Verification items for the finished model (mm, model axes). Coordinates: 2 decimals unless noted, no trailing zeros. Write each loop counter-clockwise with the first axis right and the second up, starting at its lowest first coordinate (ties: lowest second). Pieces come first, ordered by that corner, then holes. Notation, with made-up numbers: (77, -7) -> (132, -7) arc R24 ccw to (132, 26) -> close; hole circle Ø1 at (36.25, 51). An arc over 180 degrees is marked (long way). Answer in a Markdown table with one row per item.
```python
from build123d import *

# Parameters (mm, degrees)
F1_DEPTH = 12.7
F2_R     = 25.4
F3_DEPTH = 25.401


with BuildPart() as f1:
    # F0 (on Front) → F1 (new body, symmetric)
    with BuildSketch(Plane.XZ):
        with BuildLine():
            Line((952.5, 50.8), (-952.5, 50.8))
            ThreePointArc((-952.5, 50.8), (-1003.3, 0), (-952.5, -50.8))
            Line((-952.5, -50.8), (952.5, -50.8))
            ThreePointArc((952.5, -50.8), (1003.3, 0), (952.5, 50.8))
        make_face()
    extrude(amount=F1_DEPTH, both=True)

    # F2 (on face) → F3 (cut, through all)
    with BuildSketch(Plane.XZ.offset(12.7)):
        with Locations((-952.5, 0)):
            Circle(F2_R)
        with Locations((952.5, 0)):
            Circle(F2_R)
        with Locations((-317.5, 0)):
            Circle(F2_R)
    extrude(amount=-F3_DEPTH, mode=Mode.SUBTRACT)


solid = f1.part
```
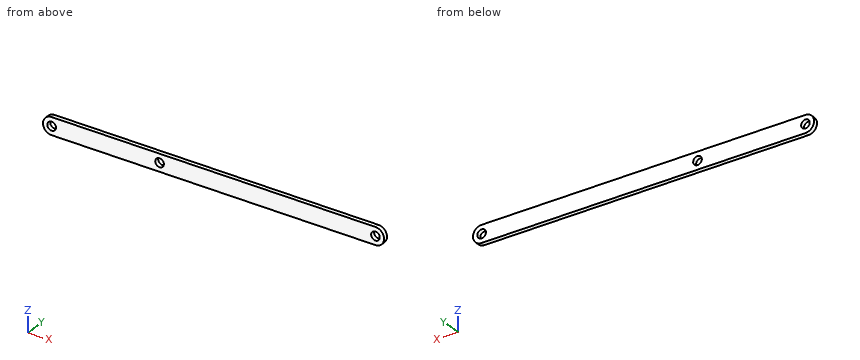
1. Thickness scan on line 1 (Z direction, x = -952.5, y = -4.5); line 2 (X direction, y = 2, z = -20); line 3 (X direction, y = 0.5, z = 23). Record the ranges inside material, lowest first. Write a range as from..to.
Geometry says:
| item | result |
|---|---|
| line 1 | -50.8..-25.4, 25.4..50.8 |
| line 2 | -999.2..-968.16, -936.84..-333.16, -301.84..936.84, 968.16..999.2 |
| line 3 | -997.8..-963.28, -941.72..-328.28, -306.72..941.72, 963.28..997.8 |
2. Depth check by flat-ended pin: P1, Ø3, axis at y = -6, z = -17.5, coming from the +X side; P2, Ø2, axis at y = 6.5, z = 15.5, coming from the +X side; P3, Ø5, axis at y = -1.5, z = 10.5, coming from the -X side. Enter the tip coordinate at first touch or a pass-through.
Geometry says:
| item | result |
|---|---|
| P1 | x = 1000.71 |
| P2 | x = 1001.19 |
| P3 | x = -1002.67 |
3. Section check A-A, the plane y = 7.75. Record the boundary of the cut face in (x, z), plus the area to 3 significant figures.
Geometry says:
| item | result |
|---|---|
| outline | (-952.5, -50.8) -> (952.5, -50.8) arc R50.8 ccw to (952.5, 50.8) -> (-952.5, 50.8) arc R50.8 ccw to start; hole circle Ø50.8 at (-952.5, 0); hole circle Ø50.8 at (-317.5, 0); hole circle Ø50.8 at (952.5, 0) |
| area | 196,000 mm^2 |
